Could you check a few things on this model? Use its own coordinates, in mm. A direction names the side the tool comes from. Round coordinates to 2 decimals unless told otherwise and drop trailing zeros. Loops run counter-clockwise (first coordinate to the right, second up) from the corner with the lowest first, then second, coordinate; pieces in that order, holes last. Notation, with made-up numbers: M 10.25,-20.75 L 48.25,-20.75 A6 cw 48.25,-12.75 Z; hole C 45,13.5 d7. An arc over 180 degrees is marked long. One line per item, written item: value. Start each with the question number.
Q1. Which directions (+Z, -Z, +X, -X, +Y, -Y) give clear straight access to the entire face, cutting with the end or side of a thin tool? Please do faces 5 (the face through (6, 12.7, 13)), 6 (the face through (11.1, 9, 4.6)), 7 (the face through (3.175, 9.3, 7.9)), 8 (the face through (4.8, 9.3, 327.025)), 9 (the face through (9.525, 7.9, 339.5)).
Q2. Please list where these lines run through material, in increasing order: line 1 along Z through (x, y) = (11.5, 6.25) (3 decimals); line 2 along Y through (x, z) = (1.95, 6.35) (3 decimals); line 3 along Z through (x, y) = (1.75, 5.5) (3 decimals).
Q3. Thinking about a two-plate mould opening in Z: for faces 1 (the face through (1.6, 9, 4.6)), 2 (the face through (6, 0, 13)), 3 (the face through (6, 6, 12.7)), 4 (the face through (1.61, 7.3, 333.52)), which applies, released by +Z, released by -Z, zero draft, split by the parting line, or undercut?
Q4. Imagine slicing it at A-A (z = 6.35). Please give me the cut outline in (x, y) (3 decimals).
Q5. I'm going to push flat-ended pins straight in: pin 1 Ø4 at (x, y) = (7, 7) entering from +Z; pin 2 Ø5 at (y, z) = (3.5, 250.5) entering from +X; pin 3 Ø1 at (x, y) = (5.5, 10) entering from -Z. Where does each tip first touch, or does it pass through?
Autodesk Inventor part; units mm, degrees
ref_plane "YZ Plane" through (0, 0, 0) normal (1, 0, 0) x (0, 1, 0)
ref_plane "XZ Plane" through (0, 0, 0) normal (0, 1, 0) x (-1, 0, 0)
ref_plane "XY Plane" through (0, 0, 0) normal (0, 0, 1) x (1, 0, 0)
sketch "Sketch1" plane through (0, 0, 0) normal (0, 0, 1) x (1, 0, 0)
  line L0 (0, 0) -> (12.7, 0)
  line L1 (12.7, 0) -> (12.7, 12.7)
  line L2 (12.7, 12.7) -> (0, 12.7)
  line L3 (0, 12.7) -> (0, 0)
  dimension "d0" = 12.7
  dimension "d1" = 12.7
extrude "Extrusion1" add sketch "Sketch1" along normal blind 342.9
sketch "Sketch2" plane through (12.7, 12.7, 342.9) normal (0, 1, 0) x (1, 0, 0)
  line L0 (-12.7, 0) -> (0, 0)
  line L1 (0, 342.9) -> (0, 0)
  line L2 (0, 342.9) -> (-12.7, 342.9)
  line L3 (-12.7, 342.9) -> (-12.7, 0)
  line L4 (-12.7, 15.875) -> (-9.525, 15.875)
  line L5 (-9.525, 15.875) -> (-9.525, 327.025)
  line L6 (-9.525, 327.025) -> (-12.7, 327.025)
  line L7 (-12.7, 327.025) -> (-12.7, 15.875)
  line L8 (0, 327.025) -> (-3.175, 327.025)
  line L9 (-3.175, 327.025) -> (-3.175, 15.875)
  line L10 (-3.175, 15.875) -> (0, 15.875)
  line L11 (0, 15.875) -> (0, 327.025)
  line L12 (-9.525, 342.9) -> (-3.175, 342.9)
  line L13 (-3.175, 342.9) -> (-3.175, 330.2)
  line L14 (-3.175, 330.2) -> (-9.525, 330.2)
  line L15 (-9.525, 330.2) -> (-9.525, 342.9)
  line L16 (-9.525, 0) -> (-3.175, 0)
  line L17 (-3.175, 0) -> (-3.175, 12.7)
  line L18 (-3.175, 12.7) -> (-9.525, 12.7)
  line L19 (-9.525, 12.7) -> (-9.525, 0)
  dimension "d4" = 15.875
  dimension "d5" = 6.35
  dimension "d6" = 15.875
  dimension "d7" = 12.7
  dimension "d8" = 12.7
extrude "Extrusion2" cut sketch "Sketch2" against normal through all contours L19 L18 L17 L0 | L3 L6 L5 L4 | L10 L9 L8 L1 | L2 L13 L14 L15
sketch "Sketch3" plane through (12.7, 0, 342.9) normal (1, 0, 0) x (0, 0, -1)
  line L0 (15.875, 12.7) -> (0, 12.7)
  line L1 (0, 12.7) -> (0, 0)
  line L2 (327.025, 12.7) -> (327.025, 0)
  line L3 (342.9, 0) -> (327.025, 0)
  line L4 (342.9, 0) -> (342.9, 12.7)
  line L5 (342.9, 12.7) -> (327.025, 12.7)
  line L6 (327.025, 0) -> (15.875, 0)
  line L7 (327.025, 12.7) -> (327.025, 0)
  line L8 (15.875, 12.7) -> (327.025, 12.7)
  line L9 (15.875, 12.7) -> (15.875, 0)
  line L10 (15.875, 12.7) -> (327.025, 12.7)
  line L11 (327.025, 12.7) -> (327.025, 9.525)
  line L12 (327.025, 9.525) -> (15.875, 9.525)
  line L13 (15.875, 9.525) -> (15.875, 12.7)
  line L14 (327.025, 3.175) -> (15.875, 3.175)
  line L15 (15.875, 3.175) -> (15.875, 0)
  line L16 (15.875, 0) -> (327.025, 0)
  line L17 (327.025, 0) -> (327.025, 3.175)
  circle A0 centre (6.35, 6.35) radius 3.175
  circle A1 centre (336.55, 6.35) radius 3.175
  point P0 (342.9, 0)
  dimension "d11" = 6.35
  dimension "d12" = 6.35
  dimension "d13" = 6.35
  dimension "d14" = 6.35
  dimension "d15" = 3.175
  dimension "d16" = 6.35
  dimension "d17" = 6.35
  dimension "d18" = 6.35
extrude "Extrusion3" cut sketch "Sketch3" against normal through all contours L2 L12 L9 L8 | L2 L6 L9 L14 | A0 | A1
fillet "Fillet1" radius 3.175 4 edges at (9.525, 9.525, 171.45) (3.175, 9.525, 171.45) (3.175, 3.175, 171.45) (9.525, 3.175, 171.45)
equation "\"d1\" = d0"
equation "\"d13\" = d12"
equation "\"d17\" = d16"
equation "\"d18\" = d17"
properties part number "8 ball manipulator piston"
Report:
1. face 5: +Z, -Z, +X, -X, +Y
1. face 6: +X, -X
1. face 7: -Z, +Y, -Y
1. face 8: none
1. face 9: +Z, +Y, -Y
2. line 1: z = 0 to 3.177, 9.523 to 15.875, 327.025 to 333.377, 339.723 to 342.9
2. line 2: y = 0 to 3.175, 9.525 to 12.7
2. line 3: z = 0 to 3.291, 9.409 to 15.875, 327.025 to 333.491, 339.609 to 342.9
3. face 1: undercut
3. face 2: zero draft
3. face 3: released by -Z
3. face 4: undercut
4. outline: M 0,0 L 3.175,0 L 3.175,3.175 L 0,3.175 Z; M 0,9.525 L 3.175,9.525 L 3.175,12.7 L 0,12.7 Z; M 9.525,0 L 12.7,0 L 12.7,3.175 L 9.525,3.175 Z; M 9.525,9.525 L 12.7,9.525 L 12.7,12.7 L 9.525,12.7 Z
5. pin 1: stops at z = 330.2
5. pin 2: stops at x = 9.51
5. pin 3: stops at z = 12.7
